Geometry check sheet. Reference: the model listing, model coordinates, mm. Face numbers are marked on the shaded views. A direction names the side the tool comes from. Coordinates: 2 decimals unless noted, no trailing zeros. Loops run counter-clockwise (first coordinate to the right, second up) from the corner with the lowest first, then second, coordinate; pieces in that order, holes last. Notation, with made-up numbers: (-35.5, -13) - (-23.5, -13) arc R20 ccw to (-23.5, 20) - close; hole circle Ø11 at (-31.5, -30). An arc over 180 degrees is marked (long way). One line per item, written item: value.
from build123d import *

# Parameters (mm, degrees)
SKETCH1_W           = 42
SKETCH1_H           = 42
SKETCH1_R           = 2.0193
SKETCH1_W_2         = 25.4
SKETCH1_H_2         = 25.4
BOSS_EXTRUDE2_DEPTH = 25.4
SKETCH17_R          = 9.525
CUT_EXTRUDE11_DEPTH = 149.304520227
SKETCH18_W          = 19.05
SKETCH18_H          = 50.8
CUT_EXTRUDE16_DEPTH = 7.62
SKETCH19_W          = 19.05
SKETCH19_H          = 50.8
CUT_EXTRUDE17_DEPTH = 7.62


with BuildPart() as part:
    # Sketch1 → Boss-Extrude2 (new body)
    with BuildSketch(Plane.XY):
        with Locations((-12.341618953, -81.761895361)):
            Rectangle(SKETCH1_W, SKETCH1_H)
        with Locations((-30.302131195, -63.801383119)):
            Circle(SKETCH1_R, mode=Mode.SUBTRACT)
        with Locations((5.618893289, -99.722407603)):
            Circle(SKETCH1_R, mode=Mode.SUBTRACT)
        with Locations((-12.341618953, -81.761895361)):
            Rectangle(SKETCH1_W_2, SKETCH1_H_2, mode=Mode.SUBTRACT)
    extrude(amount=BOSS_EXTRUDE2_DEPTH)

    # Sketch16 → Loft3 section 0
    with BuildSketch(Plane.XY.offset(25.4)):
        with BuildLine():
            Line((-33.341618953, -102.761895361), (-33.341618953, -60.761895361))
            Line((-33.341618953, -60.761895361), (8.658381047, -60.761895361))
            Line((8.658381047, -60.761895361), (8.658381047, -102.761895361))
            Line((8.658381047, -102.761895361), (-33.341618953, -102.761895361))
        make_face()
    # Sketch14 → Loft3 section 1
    with BuildSketch(Plane.XY.offset(101.6)):
        with BuildLine():
            Line((-0.231618953, -93.871895361), (-0.231618953, -69.651895361))
            Line((-0.231618953, -69.651895361), (-24.451618953, -69.651895361))
            Line((-24.451618953, -69.651895361), (-24.451618953, -93.871895361))
            Line((-24.451618953, -93.871895361), (-0.231618953, -93.871895361))
        make_face()
    loft()

    # Sketch17 → Cut-Extrude11 (cut, through all)
    with BuildSketch(Plane.XY.offset(101.6)):
        with Locations((-12.341618953, -81.761895361)):
            Circle(SKETCH17_R)
    extrude(amount=-CUT_EXTRUDE11_DEPTH, mode=Mode.SUBTRACT)

    # Sketch18 → Cut-Extrude16 (cut)
    with BuildSketch(Plane(origin=(0, -60.761895361, 0), x_dir=(1, 0, 0), z_dir=(0, 1, 0))):
        with Locations((-33.341618953, -50.8)):
            Rectangle(SKETCH18_W, SKETCH18_H)
    extrude(amount=-CUT_EXTRUDE16_DEPTH, mode=Mode.SUBTRACT)

    # Sketch19 → Cut-Extrude17 (cut)
    with BuildSketch(Plane.XZ.offset(102.761895361)):
        with Locations((8.658381047, 50.8)):
            Rectangle(SKETCH19_W, SKETCH19_H)
    extrude(amount=-CUT_EXTRUDE17_DEPTH, mode=Mode.SUBTRACT)


solid = part.part
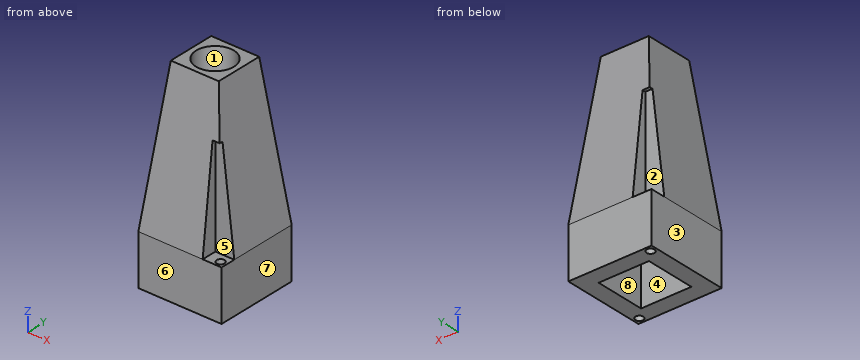
(1) Release check for a two-part mould opening along Y. For the marked faces 6, 7 and 8 record: pulls with the +Y half, pulls with the -Y half, needs draft (parallel to the pull), parting line crosses it, or undercut.
Reply:
face 6: pulls with the -Y half
face 7: needs draft
face 8: undercut
(2) Cross-section at A-A on z = 22. Record the cut outline in (x, y).
Reply:
outline: (-33.34, -102.76) - (8.66, -102.76) - (8.66, -60.76) - (-33.34, -60.76) - close; hole circle Ø4.04 at (-30.3, -63.8); hole (-25.04, -94.46) - (0.36, -94.46) - (0.36, -69.06) - (-25.04, -69.06) - close; hole circle Ø4.04 at (5.62, -99.72)
(3) Go/stop test with flat-tipped pins: pin 1 Ø1.9 at (x, y) = (1, -95.5) entering from -Z; pin 2 Ø10 at (y, z) = (-92.5, 34) entering from -X; pin 3 Ø5 at (x, z) = (-29.5, 44.5) entering from +Y; pin 4 Ø22 at (x, y) = (-12.34, -81.76) entering from -Z. Record where each tip stops, or that it passes through.
Reply:
pin 1: z = 0
pin 2: x = -32.92
pin 3: y = -68.38
pin 4: z = 25.4
(4) Material ranges on probe 1 along Y at (x, z) = (-19, 13); probe 2 along X at (y, z) = (-91.5, 17); probe 3 along X at (y, z) = (-82, 96), recorded low to high. Write a range as from..to.
Reply:
probe 1: -102.76..-94.46, -69.06..-60.76
probe 2: -33.34..-25.04, 0.36..8.66
probe 3: -25.1..-21.86, -2.82..0.42
(5) Access from +Z, -Z, +X, -X, +Y, -Y to the whole of each face (thin tool, end or side, straight path). Record for the marked faces 1, 2, 3, 4 and 5.
Reply:
face 1: +Z, -Z
face 2: -X, +Y
face 3: +Z, -Z, -X, +Y, -Y
face 4: -Z
face 5: +X, -Y
